from build123d import *

# Parameters (mm, degrees)
SKETCH1_W           = 100
SKETCH1_H           = 100
BOSS_EXTRUDE1_DEPTH = 240
SKETCH3_W           = 20
SKETCH3_H           = 100
BOSS_EXTRUDE2_DEPTH = 17.5
SKETCH4_W           = 20
SKETCH4_H           = 100
BOSS_EXTRUDE3_DEPTH = 17.5
BOSS_EXTRUDE4_DEPTH = 48.26
CUT_EXTRUDE1_DEPTH  = 20
SKETCH8_R           = 10
CUT_EXTRUDE2_DEPTH  = 60


with BuildPart() as part:
    # Sketch1 → Boss-Extrude1 (new body)
    with BuildSketch(Plane(origin=(0, 0, 0), x_dir=(0, 0, -1), z_dir=(1, 0, 0))):
        with Locations((50, 50)):
            Rectangle(SKETCH1_W, SKETCH1_H)
    extrude(amount=BOSS_EXTRUDE1_DEPTH)

    # Sketch3 → Boss-Extrude2 (add)
    with BuildSketch(Plane.XY):
        with Locations((230, 50)):
            Rectangle(SKETCH3_W, SKETCH3_H)
    extrude(amount=BOSS_EXTRUDE2_DEPTH)

    # Sketch4 → Boss-Extrude3 (add)
    with BuildSketch(Plane(origin=(0, 0, -100), x_dir=(-1, 0, 0), z_dir=(0, 0, -1))):
        with Locations((-230, 50)):
            Rectangle(SKETCH4_W, SKETCH4_H)
    extrude(amount=BOSS_EXTRUDE3_DEPTH)

    # Sketch6 → Boss-Extrude4 (add)
    with BuildSketch(Plane(origin=(240, 0, 0), x_dir=(0, 0, -1), z_dir=(1, 0, 0))):
        with BuildLine():
            ThreePointArc((65.9, 50), (61.242997821, 61.242997821), (50, 65.9))
            Line((50, 65.9), (50, 50))
            Line((50, 50), (34.1, 50))
            ThreePointArc((34.1, 50), (50, 34.1), (65.9, 50))
        make_face()
        with BuildLine():
            Line((50, 50), (50, 65.9))
            ThreePointArc((50, 65.9), (38.757002179, 61.242997821), (34.1, 50))
            Line((34.1, 50), (50, 50))
        make_face()
    extrude(amount=BOSS_EXTRUDE4_DEPTH)

    # Sketch7 → Cut-Extrude1 (cut)
    with BuildSketch(Plane(origin=(240, 0, 0), x_dir=(0, 0, -1), z_dir=(1, 0, 0))):
        with BuildLine():
            Line((0, 63.65), (0, 70))
            Line((0, 70), (6.35, 70))
            ThreePointArc((6.35, 70), (-4.490128061, 74.490128061), (0, 63.65))
        make_face()
        with BuildLine():
            Line((6.35, 70), (0, 70))
            Line((0, 70), (0, 63.65))
            ThreePointArc((0, 63.65), (4.490128061, 65.509871939), (6.35, 70))
        make_face()
        with BuildLine():
            ThreePointArc((6.35, 30), (4.490128061, 34.490128061), (0, 36.35))
            Line((0, 36.35), (0, 30))
            Line((0, 30), (6.35, 30))
        make_face()
        with BuildLine():
            Line((0, 30), (0, 36.35))
            ThreePointArc((0, 36.35), (-4.490128061, 25.509871939), (6.35, 30))
            Line((6.35, 30), (0, 30))
        make_face()
        with BuildLine():
            ThreePointArc((106.35, 30), (104.490128061, 34.490128061), (100, 36.35))
            Line((100, 36.35), (100, 30))
            Line((100, 30), (93.65, 30))
            ThreePointArc((93.65, 30), (100, 23.65), (106.35, 30))
        make_face()
        with BuildLine():
            Line((100, 30), (100, 36.35))
            ThreePointArc((100, 36.35), (95.509871939, 34.490128061), (93.65, 30))
            Line((93.65, 30), (100, 30))
        make_face()
        with BuildLine():
            ThreePointArc((106.35, 70), (100, 76.35), (93.65, 70))
            Line((93.65, 70), (100, 70))
            Line((100, 70), (100, 63.65))
            ThreePointArc((100, 63.65), (104.490128061, 65.509871939), (106.35, 70))
        make_face()
        with BuildLine():
            Line((100, 70), (93.65, 70))
            ThreePointArc((93.65, 70), (95.509871939, 65.509871939), (100, 63.65))
            Line((100, 63.65), (100, 70))
        make_face()
    extrude(amount=-CUT_EXTRUDE1_DEPTH, mode=Mode.SUBTRACT)

    # Sketch8 → Cut-Extrude2 (cut)
    with BuildSketch(Plane.ZY.offset(-220)):
        with Locations((0, 70)):
            Circle(SKETCH8_R)
        with Locations((0, 30)):
            Circle(SKETCH8_R)
        with Locations((-100, 70)):
            Circle(SKETCH8_R)
        with Locations((-100, 30)):
            Circle(SKETCH8_R)
    extrude(amount=CUT_EXTRUDE2_DEPTH, mode=Mode.SUBTRACT)


solid = part.part
Build history of the part. All positions in model axes, mm. A direction names the side the tool comes from. Round coordinates to 2 decimals unless told otherwise and drop trailing zeros. Loops run counter-clockwise (first coordinate to the right, second up) from the corner with the lowest first, then second, coordinate; pieces in that order, holes last. Notation, with made-up numbers: (41.5, 41) -> (64.5, 41) arc R20 cw to (64.5, 80) -> close; hole circle Ø5 at (81, 43). An arc over 180 degrees is marked (long way). One line per item, written item: value. Start each with the question number.
Q1. Cut at B-B on x = 209. List the corners of the cut face in (y, z), plus the area to 3 significant figures.
Q2. Two-plate mould, pull along Y, no slides. Class faces 1 (the face through (122, 0, -49)), 2 (the face through (240, 38, -64)), 3 (the face through (190, 70, -10)): released by +Y, released by -Y, zero draft, split by the parting line, or undercut.
Q3. Drop flat-ended pins along their axis: pin 1 Ø11.5 at (y, z) = (70, 0) entering from +X; pin 2 Ø10 at (y, z) = (14.5, -63) entering from -X; pin 3 Ø8 at (y, z) = (41.5, 10) entering from -X; pin 4 Ø5 at (y, z) = (32, -94) entering from +X. Give the stop position or say it passes through.
Q4. Cut at C-C on y = 86.5. List the corners of the cut face in (x, z), plus the area to 3 significant figures.
Q5. 3-axis set-ups, long thin cutter, end or side, ignore diameter. For faces 4 (the face through (108, 49, -100)), 5 (the face through (160, 30, -4)), 6 (the face through (160, 30, -96)): which of +Z, -Z, +X, -X, +Y, -Y reach the whole face in a straight line?
Q6. Probe line 1 along Y through (x, z) = (234.5, 0); line 2 along Z through (x, y) = (226, 30); line 3 along X through (y, z) = (46.5, -86). List the from-to ranges inside material, lowest first.
Q7. Cut at D-D on z = -81.5. List the corners of the cut face in (x, y), plus the area to 3 significant figures.
Q8. Cut at A-A on y = 27. List the corners of the cut face in (x, z), plus the area to 3 significant figures.
Computed:
1. outline: (0, -100) -> (20, -100) arc R10 cw to (40, -100) -> (60, -100) arc R10 cw to (80, -100) -> (100, -100) -> (100, 0) -> (80, 0) arc R10 cw to (60, 0) -> (40, 0) arc R10 cw to (20, 0) -> (0, 0) -> close
1. area: 9,370 mm²
2. face 1: released by -Y
2. face 2: zero draft
2. face 3: undercut
3. pin 1: x = 160
3. pin 2: x = 0
3. pin 3: x = 220
3. pin 4: x = 240
4. outline: (0, -100) -> (220, -100) -> (220, -117.5) -> (240, -117.5) -> (240, 17.5) -> (220, 17.5) -> (220, 0) -> (0, 0) -> close
4. area: 24,700 mm²
5. face 4: -Z, -X, +Y, -Y
5. face 5: +Z
5. face 6: -Z
6. line 1: 0 to 23.65, 36.35 to 63.65, 76.35 to 100
6. line 2: -117.5 to -106.35, -93.65 to -6.35, 6.35 to 17.5
6. line 3: 0 to 240
7. outline: (0, 0) -> (240, 0) -> (240, 100) -> (0, 100) -> close
7. area: 24,000 mm²
8. outline: (0, -100) -> (160, -100) -> (160, -90.46) -> (220, -90.46) -> (220, -94.4) -> (240, -94.4) -> (240, -5.6) -> (220, -5.6) -> (220, -9.54) -> (160, -9.54) -> (160, 0) -> (0, 0) -> close; (220, -117.5) -> (240, -117.5) -> (240, -105.6) -> (220, -105.6) -> close; (220, 5.6) -> (240, 5.6) -> (240, 17.5) -> (220, 17.5) -> close
8. area: 23,100 mm²
